Geometry: final body of the model. Coordinates: model frame, mm. A direction names the side the tool comes from. Give positions to 0.01 mm unless a question says otherwise; leave off trailing zeros. Loops run counter-clockwise (first coordinate to the right, second up) from the corner with the lowest first, then second, coordinate; pieces in that order, holes last. Notation, with made-up numbers: (87.5, 57) -> (121.5, 57) arc R16 ccw to (121.5, 85) -> close; hole circle Ø2 at (11, 84). An arc over 180 degrees is marked (long way). One line per question, with ' | ' between items. Start each with the question number.
Item 1: Section C-C on x = -170.5. Return loops of the section in (y, z).
Item 2: Material intervals for line 1 along Z through (x, y) = (-138, -110); line 2 along X through (y, z) = (-76, 8); line 3 along Y through (x, z) = (-101, 20.5), sorted ascending. Write a range as [from, to].
Item 3: Section B-B on y = -43. Return loops of the section in (x, z).
Item 4: Set-up query: faces 5 (the flat face through (-200, -2, 25)), 6 (the flat face through (-197, -1, 25)), 7 (the flat face through (3, -122, 25)). Return all of +Z, -Z, +X, -X, +Y, -Y with unobstructed straight access to the full face (end or side cutting, diameter ignored); none if empty.
Item 5: Mould query, pull axis Z, two halves, no side actions, for faces 1 (the flat face through (3, 125, 25)), 2 (the flat face through (3, 122, 25)), 3 (the flat face through (-1, 102, 0)), 4 (the flat face through (-1, 102, 50)). Classes: released by +Z, released by -Z, zero draft, split by the parting line, or undercut.
Item 6: Section A-A on z = 24. Return loops of the section in (x, y), then the cut area to 3 significant figures.
from build123d import *

# Parameters (mm, degrees)
F0_W     = 400
F0_H     = 250
F0_W_2   = 350
F0_H_2   = 200
F1_DEPTH = 50
F2_W     = 25
F2_H     = 44
F3_DEPTH = 250
F4_W     = 25
F4_H     = 44
F5_DEPTH = 400
F6_DEPTH = 25
F7_DEPTH = 25
F8_DEPTH = 25
F9_DEPTH = 25


with BuildPart() as f1:
    # F0 (on Top) → F1 (new body)
    with BuildSketch(Plane.XY):
        Rectangle(F0_W, F0_H)
        Rectangle(F0_W_2, F0_H_2, mode=Mode.SUBTRACT)
    extrude(amount=F1_DEPTH)

    # F2 (on face) → F3 (cut, through all)
    with BuildSketch(Plane.XZ.offset(125)):
        with Locations((184.5, 25)):
            Rectangle(F2_W, F2_H)
        with Locations((-184.5, 25)):
            Rectangle(F2_W, F2_H)
    extrude(amount=-F3_DEPTH, mode=Mode.SUBTRACT)

    # F4 (on face) → F5 (cut, through all)
    with BuildSketch(Plane.YZ.offset(200)):
        with Locations((109.5, 25)):
            Rectangle(F4_W, F4_H)
        with Locations((-109.5, 25)):
            Rectangle(F4_W, F4_H)
    extrude(amount=-F5_DEPTH, mode=Mode.SUBTRACT)

    # F6 (add): a face of the model
    f6_faces = [f1.faces().sort_by_distance(p)[0] for p in [
        (172, -123.5, 25),
    ]]
    extrude(f6_faces, amount=F6_DEPTH)

    # F7 (add): a face of the model
    f7_faces = [f1.faces().sort_by_distance(p)[0] for p in [
        (172, 123.5, 25),
    ]]
    extrude(f7_faces, amount=F7_DEPTH)

    # F8 (add): a face of the model
    f8_faces = [f1.faces().sort_by_distance(p)[0] for p in [
        (-172, 123.5, 25),
    ]]
    extrude(f8_faces, amount=F8_DEPTH)

    # F9 (add): a face of the model
    f9_faces = [f1.faces().sort_by_distance(p)[0] for p in [
        (-172, -123.5, 25),
    ]]
    extrude(f9_faces, amount=F9_DEPTH)


solid = f1.part
Result sheet:
1) outline: (-125, 0) -> (-100, 0) -> (-100, 3) -> (-122, 3) -> (-122, 47) -> (-100, 47) -> (-100, 50) -> (-125, 50) -> close; (100, 0) -> (125, 0) -> (125, 50) -> (100, 50) -> (100, 47) -> (122, 47) -> (122, 3) -> (100, 3) -> close
2) line 1: z = [0, 3], [47, 50] | line 2: x = [-200, -197], [197, 200] | line 3: y = [-125, -122], [122, 125]
3) outline: (-200, 0) -> (-175, 0) -> (-175, 3) -> (-197, 3) -> (-197, 47) -> (-175, 47) -> (-175, 50) -> (-200, 50) -> close; (175, 0) -> (200, 0) -> (200, 50) -> (175, 50) -> (175, 47) -> (197, 47) -> (197, 3) -> (175, 3) -> close
4) face 5: +Z, -Z, -X, +Y, -Y | face 6: none | face 7: +X, -X
5) face 1: zero draft | face 2: undercut | face 3: released by -Z | face 4: released by +Z
6) outline: (-200, -125) -> (200, -125) -> (200, -122) -> (-200, -122) -> close; (-200, -97) -> (-197, -97) -> (-197, 97) -> (-200, 97) -> close; (-200, 122) -> (200, 122) -> (200, 125) -> (-200, 125) -> close; (197, -97) -> (200, -97) -> (200, 97) -> (197, 97) -> close | area: 3,560 mm²
